Geometry: see drawing. Coordinates: mm, zero at the bounding-box minimum. A direction names the side the tool comes from. Coordinates: 2 decimals unless noted, no trailing zeros. Write each loop counter-clockwise with the first axis right and the second up, starting at its lowest first coordinate (ties: lowest second). Pieces come first, ordered by that corner, then holes. Notation, with made-up numbers: (-3, 43.5) - (39, 43.5) arc R10 cw to (39, 59.5) - close; hole circle Ø8 at (84.5, -38). An arc over 180 degrees is marked (long way). One line per question, with ' | ' between items. Start each with the question number.
Q1. Contact query for flat-ended pins moving along their axis: P1, Ø6, axis at y = 230, z = 4.5, coming from the +X side; P2, Ø11, axis at x = 204.5, z = 14.5, coming from the +Y side. Output: stop coordinate, or through.
Q2. Cut plane A-A, the plane z = 17.5. Return loops of the section in (x, y).
Q3. Access query for the marked faces 1 and 2. Directions: +Z, -Z, +X, -X, +Y, -Y. A direction counts if a zero-diameter tool reaches every point of the face in a straight line with its end or side. Return the directions, or none.
Q4. Line query: line 1 (X direction, y = 273.5, z = 3). Output: solid intervals per line, ascending.
Q5. Cut plane B-B, the plane y = 241.5. Return loops of the section in (x, z).
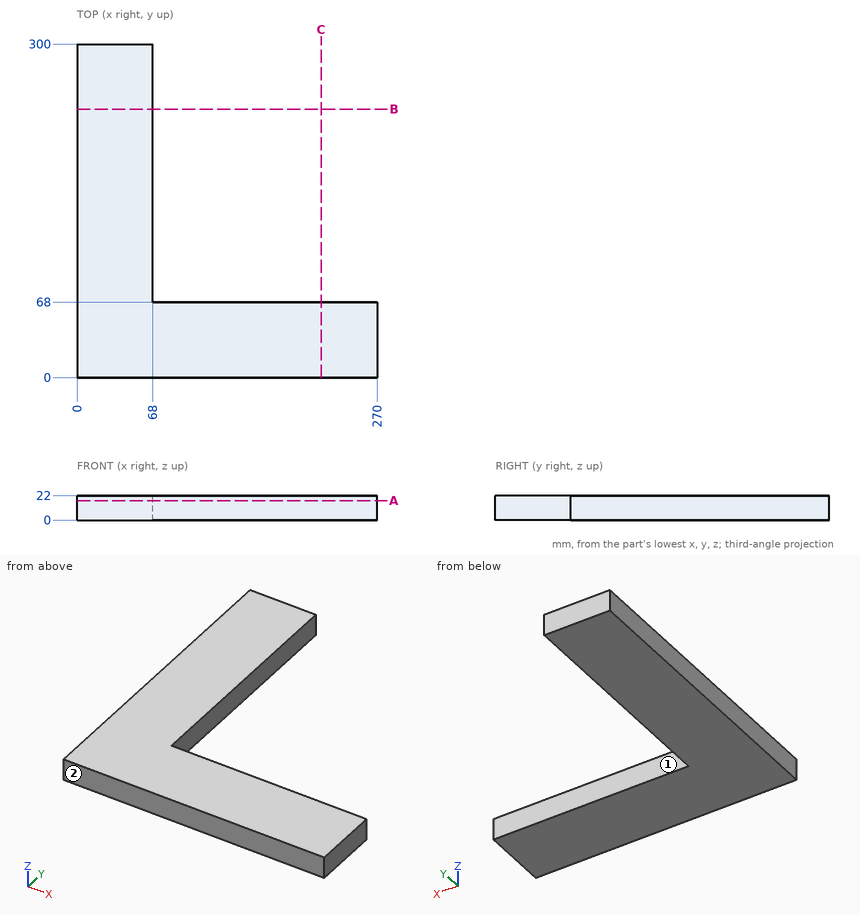
Reply:
1) P1: stops at x = 68 | P2: stops at y = 68
2) outline: (0, 0) - (270, 0) - (270, 68) - (68, 68) - (68, 300) - (0, 300) - close
3) face 1: +Z, -Z, +X, +Y | face 2: +Z, -Z, +X, -X, -Y
4) line 1: x = 0 to 68
5) outline: (0, 0) - (68, 0) - (68, 22) - (0, 22) - close
